from build123d import *

# Parameters (mm, degrees)
SKETCH2_R                = 0.5
CUT_EXTRUDE2_DEPTH       = 18.207691702
SKETCH5_W                = 5
SKETCH5_H                = 18
CUT_EXTRUDE4_DEPTH       = 20
REVOLVE3_ANGLE           = 90
REVOLVE3_OTHER_WAY_ANGLE = 90
SKETCH12_W               = 15.157920946
SKETCH12_H               = 18.962900337
CUT_EXTRUDE5_DEPTH       = 9
SKETCH14_R               = 0.5
CUT_EXTRUDE6_DEPTH       = 6
SKETCH15_R               = 0.75
CUT_EXTRUDE7_DEPTH       = 7


with BuildPart() as part:
    # Sketch1 → Revolve1 (revolve)
    with BuildSketch(Plane.XY):
        with BuildLine():
            Line((4.88, 0), (6.88, 0))
            add(Edge.make_bspline(
                [(6.88, 0), (6.476901655, 3.177692832), (5.808868292, 8.357754247), (4.378289276, 15.464596201), (1.111060579, 17.280233516), (0, 17.2)],
                knots=[0, 0, 0, 0, 0.473754928, 0.838492431, 1, 1, 1, 1], degree=3))
            Line((0, 17.2), (0, 15.4))
            add(Edge.make_bspline(
                [(0, 15.4), (1.563029619, 15.297760208), (2.284243197, 13.63319745)],
                knots=[0, 0, 0, 1, 1, 1], degree=2))
            add(Edge.make_bspline(
                [(2.284243197, 13.63319745), (4.266259497, 7.778351244), (4.88, 1.606249126)],
                knots=[0, 0, 0, 1, 1, 1], degree=2))
            ThreePointArc((4.88, 1.606249126), (4.905839008, 0.803124563), (4.88, 0))
        make_face()
    revolve(axis=Axis((0, 18.057905706, 0), (0, -1, 0)))

    # Sketch2 → Cut-Extrude2 (cut, through all)
    with BuildSketch(Plane(origin=(0, 0, 0), x_dir=(1, 0, 0), z_dir=(0, 1, 0))):
        Circle(SKETCH2_R)
    extrude(amount=CUT_EXTRUDE2_DEPTH, mode=Mode.SUBTRACT)

    # Sketch5 → Cut-Extrude4 (cut)
    with BuildSketch(Plane.XZ):
        with Locations((4.5, 0.912005105)):
            Rectangle(SKETCH5_W, SKETCH5_H)
    extrude(amount=-CUT_EXTRUDE4_DEPTH, mode=Mode.SUBTRACT)

    # Sketch9 → Revolve3 (revolve)
    with BuildSketch(Plane.XY):
        with BuildLine():
            Line((0, 17.2), (0, 0))
            Line((0, 0), (4.88, 0))
            Line((4.88, 0), (6.88, 0))
            add(Edge.make_bspline(
                [(6.88, 0), (6.476901655, 3.177692832), (5.808868292, 8.357754247), (4.378289276, 15.464596201), (1.111060579, 17.280233516), (0, 17.2)],
                knots=[0, 0, 0, 0, 0.473754928, 0.838492431, 1, 1, 1, 1], degree=3))
        make_face()
    revolve(axis=Axis((0, 17.2, 0), (0, -1, 0)), revolution_arc=REVOLVE3_ANGLE)

    # Sketch9 → Revolve3 other way (revolve)
    with BuildSketch(Plane.XY):
        with BuildLine():
            Line((0, 17.2), (0, 0))
            Line((0, 0), (4.88, 0))
            Line((4.88, 0), (6.88, 0))
            add(Edge.make_bspline(
                [(6.88, 0), (6.476901655, 3.177692832), (5.808868292, 8.357754247), (4.378289276, 15.464596201), (1.111060579, 17.280233516), (0, 17.2)],
                knots=[0, 0, 0, 0, 0.473754928, 0.838492431, 1, 1, 1, 1], degree=3))
        make_face()
    revolve(axis=Axis((0, 17.2, 0), (0, 1, 0)), revolution_arc=REVOLVE3_OTHER_WAY_ANGLE)

    # Sketch12 → Cut-Extrude5 (cut)
    with BuildSketch(Plane(origin=(10, 0, 0), x_dir=(0, 0, -1), z_dir=(1, 0, 0))):
        with Locations((0, 8.631516603)):
            Rectangle(SKETCH12_W, SKETCH12_H)
    extrude(amount=-CUT_EXTRUDE5_DEPTH, mode=Mode.SUBTRACT)

    # Sketch14 → Cut-Extrude6 (cut)
    with BuildSketch(Plane(origin=(0, 20, 0), x_dir=(1, 0, 0), z_dir=(0, 1, 0))):
        Circle(SKETCH14_R)
    extrude(amount=-CUT_EXTRUDE6_DEPTH, mode=Mode.SUBTRACT)

    # Sketch15 → Cut-Extrude7 (cut)
    with BuildSketch(Plane(origin=(0, 20, 0), x_dir=(1, 0, 0), z_dir=(0, 1, 0))):
        Circle(SKETCH15_R)
    extrude(amount=-CUT_EXTRUDE7_DEPTH, mode=Mode.SUBTRACT)


solid = part.part
Can you work these out from the model? Positions are in its coordinate system, mm. Coordinates: 2 decimals unless noted, no trailing zeros. Answer as a JSON object with one key per item and string values. Group by question number.
Item 1: If I drill on L1, parallel to Z at x = 0, y = 15.35; L2, parallel to Z at x = 0, y = 15.5; L3, parallel to X at y = 1.75, z = 0.75, over which ranges is the centre line in solid material (lowest first)? Write a range as from..to.
Item 2: For pin 1 (3 mm diameter, centred on y = 9, z = -2, fed in from -X); pin 2 (5 mm diameter, centred on y = 12, z = -3, fed in from +X); pin 3 (1 mm diameter, centred on y = 10, z = -0.5, fed in from -X); pin 4 (8 mm diameter, centred on x = 5.5, z = 3, fed in from -Y), each with a flat end and sliding along its axis, tell me the tip position at first contact or that it passes through.
Item 3: If we mould it in two halves opening along Z, with no side actions, what happens to faces 1 (the face through (-5, 0, -2)), 2 (the face through (0, 6, 0)), 3 (the face through (0.69, 15.57, 0.29))? For each: released by +Z, released by -Z, zero draft, split by the parting line, or undercut.
Returned:
{
 "1": {"L1": "z = -3.45..-0.75, 0.75..3.45", "L2": "z = -3.33..-0.75, 0.75..3.33", "L3": "x = -6.61..-4.81, 0..1"},
 "2": {"pin 1": "stops at x = -5.7", "pin 2": "stops at x = 1", "pin 3": "stops at x = -5.5", "pin 4": "passes through"},
 "3": {"face 1": "zero draft", "face 2": "undercut", "face 3": "undercut"}
}
